Could you check a few things on this drawing? It's one solid part, dimensions in mm from its lowest x, y, z. A direction names the side the tool comes from. Give positions to 0.01 mm unless a question says otherwise; leave off trailing zeros. Order: outer loops, then holes, each group sorted by start corner. A loop starts at its lowest first (then second) coordinate and runs counter-clockwise, first axis right, second up. Notation, with made-up numbers: (42.25, 88) -> (58.25, 88) arc R37 cw to (58.25, 126) -> close; hole circle Ø8 at (82.5, -2.5). An arc over 180 degrees is marked (long way). Write each question's results on one line, items separated by ' | '. Start each with the question number.
Q1. I need wall thicknesses on line 1 along Y through (x, z) = (28, 7); line 2 along X through (y, z) = (23.5, 36); line 3 along Y through (x, z) = (27.5, 39.5). Which ranges of each line are inside material? Lowest first, please. Write a range as [from, to].
Q2. Thinking about a two-plate mould opening in X: for the marked faces 3, 4 and 5, which applies, pulls with the +X half, pulls with the -X half, needs draft (parallel to the pull), parting line crosses it, or undercut?
Q3. Imagine slicing it at A-A, the plane x = 28. Please give me the cut outline in (y, z).
Q4. For the marked faces 1 and 2, which set-ups out of +Z, -Z, +X, -X, +Y, -Y let a thin tool reach every point of the face, with its end or its side?
Q5. I'm going to push flat-ended pins straight in: pin 1 (2 mm diameter, centred on x = 11, z = 32.5, fed in from -Y); pin 2 (3 mm diameter, centred on x = 34, z = 30, fed in from +Y); pin 3 (2.5 mm diameter, centred on x = 28, y = 45.5, fed in from -Z); pin 4 (5 mm diameter, centred on x = 50.5, y = 23, fed in from +Z). Where does each tip first touch, or does it pass through?
Q6. Imagine slicing it at D-D, the plane x = 42. Please give me the cut outline in (y, z), then the cut area to 3 significant figures.
Q7. Imagine slicing it at C-C, the plane z = 27.5. Please give me the cut outline in (x, y).
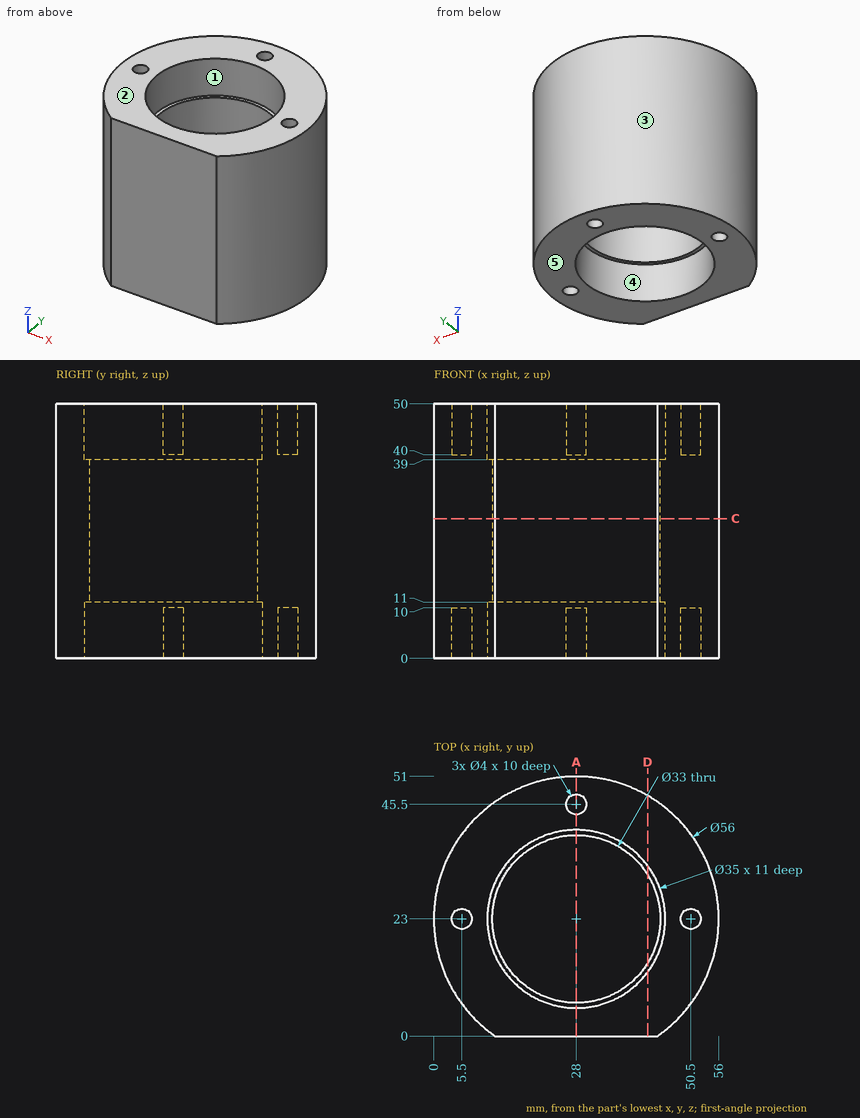
Geometry check:
1) line 1: [0, 5.5], [40.5, 43.5], [47.5, 51] | line 2: [0, 11.51], [44.49, 56] | line 3: [0, 5.51], [40.49, 51]
2) face 3: parting line crosses it | face 4: undercut | face 5: needs draft
3) outline: (0, 0) -> (5.5, 0) -> (5.5, 11) -> (6.5, 11) -> (6.5, 39) -> (5.5, 39) -> (5.5, 50) -> (0, 50) -> close; (39.5, 11) -> (40.5, 11) -> (40.5, 0) -> (43.5, 0) -> (43.5, 10) -> (47.5, 10) -> (47.5, 0) -> (51, 0) -> (51, 50) -> (47.5, 50) -> (47.5, 40) -> (43.5, 40) -> (43.5, 50) -> (40.5, 50) -> (40.5, 39) -> (39.5, 39) -> close
4) face 1: +Z | face 2: +Z, +X, -X, +Y, -Y
5) pin 1: y = 0.02 | pin 2: y = 50.64 | pin 3: z = 10 | pin 4: z = 50
6) outline: (0, 0) -> (12.5, 0) -> (12.5, 11) -> (14.27, 11) -> (14.27, 39) -> (12.5, 39) -> (12.5, 50) -> (0, 50) -> close; (31.73, 11) -> (33.5, 11) -> (33.5, 0) -> (47.25, 0) -> (47.25, 50) -> (33.5, 50) -> (33.5, 39) -> (31.73, 39) -> close | area: 1,410 mm²
7) outline: (12.03, 0) -> (43.97, 0) arc R28 ccw (long way) to start; hole circle Ø33 at (28, 23)
